```python
from build123d import *

# Parameters (mm, degrees)
ESQUISSE1_W             = 130
ESQUISSE1_H             = 80
BOSS_EXTRU_1_DEPTH      = 2
ESQUISSE2_W             = 130
ESQUISSE2_H             = 80
ESQUISSE2_R             = 5.1
BOSS_EXTRU_2_DEPTH      = 32.7
ESQUISSE3_R             = 2.5
ESQUISSE3_W             = 14
ESQUISSE3_H             = 7.5
ENL_V_MAT_EXTRU_1_DEPTH = 10
ESQUISSE4_R             = 5.5
BOSS_EXTRU_3_DEPTH      = 29.5


with BuildPart() as part:
    # Esquisse1 → Boss.-Extru.1 (new body)
    with BuildSketch(Plane(origin=(0, 0, 0), x_dir=(1, 0, 0), z_dir=(0, 1, 0))):
        with Locations((65, 40)):
            Rectangle(ESQUISSE1_W, ESQUISSE1_H)
    extrude(amount=BOSS_EXTRU_1_DEPTH)

    # Esquisse2 → Boss.-Extru.2 (add)
    with BuildSketch(Plane.XZ):
        with Locations((65, -40)):
            Rectangle(ESQUISSE2_W, ESQUISSE2_H)
        with Locations((123, -7)):
            Circle(ESQUISSE2_R, mode=Mode.SUBTRACT)
        with Locations((123, -73)):
            Circle(ESQUISSE2_R, mode=Mode.SUBTRACT)
        with Locations((7, -7)):
            Circle(ESQUISSE2_R, mode=Mode.SUBTRACT)
        with Locations((7, -73)):
            Circle(ESQUISSE2_R, mode=Mode.SUBTRACT)
        with BuildLine():
            Line((11.898979486, -78), (118.101020514, -78))
            ThreePointArc((118.101020514, -78), (118.050252532, -68.050252532), (128, -68.101020514))
            Line((128, -68.101020514), (128, -11.898979486))
            ThreePointArc((128, -11.898979486), (118.050252532, -11.949747468), (118.101020514, -2))
            Line((118.101020514, -2), (11.898979486, -2))
            ThreePointArc((11.898979486, -2), (11.949747468, -11.949747468), (2, -11.898979486))
            Line((2, -11.898979486), (2, -68.101020514))
            ThreePointArc((2, -68.101020514), (11.949747468, -68.050252532), (11.898979486, -78))
        make_face(mode=Mode.SUBTRACT)
    extrude(amount=BOSS_EXTRU_2_DEPTH)

    # Esquisse3 → Enlèv. mat.-Extru.1 (cut)
    with BuildSketch(Plane(origin=(130, 0, 0), x_dir=(0, 0, -1), z_dir=(1, 0, 0))):
        with Locations((39, -8)):
            Circle(ESQUISSE3_R)
        with Locations((46, -8)):
            Circle(ESQUISSE3_R)
        with Locations((53, -8)):
            Circle(ESQUISSE3_R)
        with Locations((60, -8)):
            Circle(ESQUISSE3_R)
        with Locations((25, -9.75)):
            Rectangle(ESQUISSE3_W, ESQUISSE3_H)
    extrude(amount=-ENL_V_MAT_EXTRU_1_DEPTH, mode=Mode.SUBTRACT)

    # Esquisse4 → Boss.-Extru.3 (add)
    with BuildSketch(Plane.XZ):
        with Locations((7, -7)):
            Circle(ESQUISSE4_R)
        with Locations((123, -7)):
            Circle(ESQUISSE4_R)
        with Locations((123, -73)):
            Circle(ESQUISSE4_R)
        with Locations((7, -73)):
            Circle(ESQUISSE4_R)
    extrude(amount=BOSS_EXTRU_3_DEPTH)


solid = part.part
```
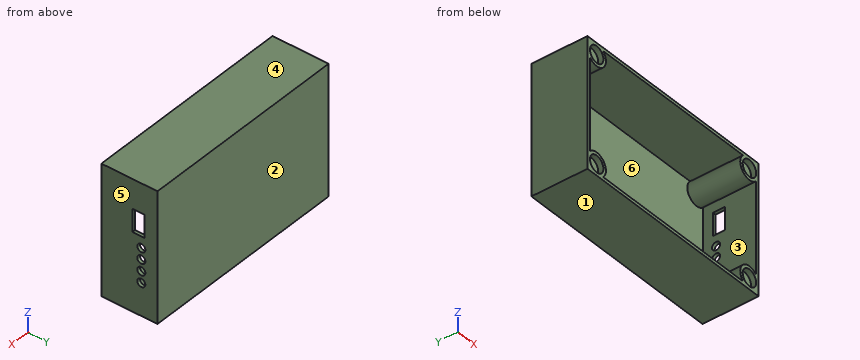
Work out the finished part from the listing and answer in its coordinate system (mm). Face numbers are marked on the shaded views. A direction names the side the tool comes from. Round coordinates to 2 decimals unless told otherwise and drop trailing zeros. Loops run counter-clockwise (first coordinate to the right, second up) from the corner with the lowest first, then second, coordinate; pieces in that order, holes last. Notation, with made-up numbers: M 22,72 L 57,72 A13 ccw 57,89 Z; hole C 0,46 d10. An arc over 180 degrees is marked long. One line per question, with ' | ' between items.
Q1. Find section D-D, the plane z = -30. Give the vertices of the cut face in (x, y).
Conclusion:
outline: M 0,-32.7 L 2,-32.7 L 2,0 L 128,0 L 128,-6 L 130,-6 L 130,2 L 0,2 Z; M 128,-32.7 L 130,-32.7 L 130,-13.5 L 128,-13.5 Z
Q2. Find section A-A, the plane z = -53. Give the vertices of the cut face in (x, y), then the cut area to 3 significant figures.
Conclusion:
outline: M 0,-32.7 L 2,-32.7 L 2,0 L 128,0 L 128,-5.5 L 130,-5.5 L 130,2 L 0,2 Z; M 128,-32.7 L 130,-32.7 L 130,-10.5 L 128,-10.5 Z | area: 381 mm2
Q3. Each of these flat-tipped pins is pushed along its axis until it touches: pin 1 Ø4 at (y, z) = (-8, -53) entering from +X; pin 2 Ø5 at (x, z) = (6, -6.5) entering from -Y; pin 3 Ø23 at (x, z) = (93, -24) entering from -Y. Where does it stop, or does it pass through?
Conclusion:
pin 1: stops at x = 2 | pin 2: stops at y = -29.5 | pin 3: stops at y = 0
Q4. Find section B-B, the plane y = -19. Give the vertices of the cut face in (x, z).
Conclusion:
outline: M 0,-80 L 130,-80 L 130,0 L 0,0 Z; hole M 2,-68.1 A7 cw long 11.9,-78 L 118.1,-78 A7 cw long 128,-68.1 L 128,-11.9 A7 cw long 118.1,-2 L 11.9,-2 A7 cw long 2,-11.9 Z
Q5. Consider line 1 along Z through (x, y) = (66.5, -15.5); line 2 along X through (y, z) = (-25, -38); line 3 along Z through (x, y) = (7, -31.3). Determine where each line is inside the solid, lowest interval first. Write a range as from..to.
Conclusion:
line 1: z = -80..-78, -2..0 | line 2: x = 0..2, 128..130 | line 3: z = -80..-78.1, -67.9..-66, -14..-12.1, -1.9..0
Q6. The mould has two halves that part along Z. Classify the marked faces 1, 2, 3 and 4: +Z half, -Z half, draft (parallel to the pull), parting line (faces both ways), or undercut.
Conclusion:
face 1: -Z half | face 2: draft | face 3: undercut | face 4: +Z half
Q7. A tool of negligible diameter and unlimited length cuts with its end or side. For the marked faces 5 and 6, from which of +Z, -Z, +X, -X, +Y, -Y can it reach the whole face along a straight path? Write none if from no direction.
Conclusion:
face 5: +Z, -Z, +X, +Y, -Y | face 6: -Y
Q8. Find section C-C, the plane x = 51. Give the vertices of the cut face in (y, z).
Conclusion:
outline: M -32.7,-80 L 2,-80 L 2,0 L -32.7,0 L -32.7,-2 L 0,-2 L 0,-78 L -32.7,-78 Z
